Input: dimensioned drawing with shaded views. Units: mm. Origin: part minimum x, y, z. Give positions to 0.01 mm unless a question says otherwise; leave off trailing zeros. Order: outer loops, then holes, each group sorted by start corner. A loop starts at its lowest first (then second) coordinate and runs counter-clockwise, first axis right, second up.
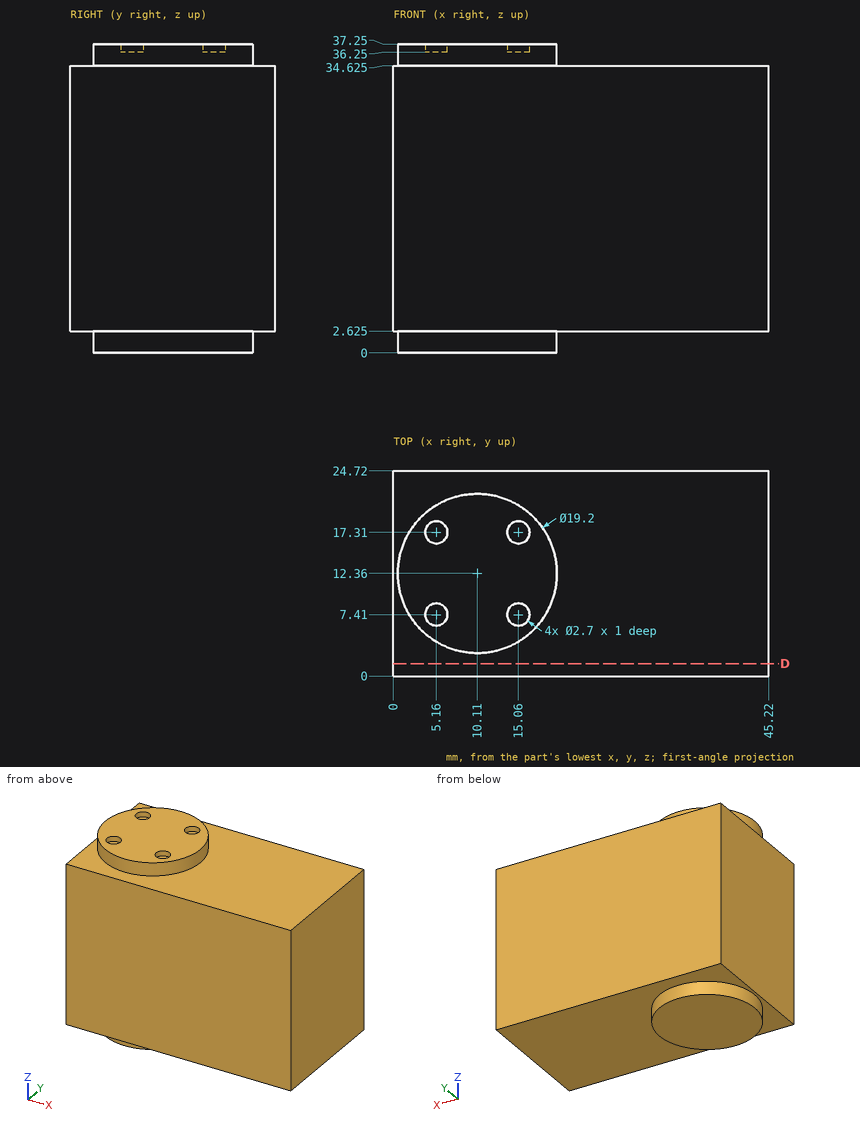
1) First-contact query: P1, Ø2, axis at x = 15.06, y = 17.31, coming from the +Z side; P2, Ø1.3, axis at x = 4.5, y = 16.5, coming from the +Z side; P3, Ø4, axis at x = 33.5, y = 18, coming from the -Z side (3 decimals); P4, Ø6, axis at x = 29.5, y = 10.5, coming from the +Z side (3 decimals). Flat tips, straight axial feed; report the tip coordinate or a pass-through.
2) Cut plane D-D (y = 1.5). Return the cut outline in (x, z) (1 decimal).
3) Line query: probe 1 along Z at (x, y) = (19.5, 9) (1 decimal); probe 2 along Y at (x, z) = (2, 35) (1 decimal); probe 3 along X at (y, z) = (15.75, 35). Output: solid intervals per line, ascending.
Geometry says:
1. P1: stops at z = 36.25
1. P2: stops at z = 37.25
1. P3: stops at z = 2.625
1. P4: stops at z = 34.625
2. outline: (0, 2.6) - (45.2, 2.6) - (45.2, 34.6) - (0, 34.6) - close
3. probe 1: z = 2.6 to 34.6
3. probe 2: y = 7.2 to 17.5
3. probe 3: x = 1.13 to 19.09
